The listing builds one solid part. Answer for the finished solid, in the listing's coordinates (mm). A direction names the side the tool comes from. Coordinates: 2 decimals unless noted, no trailing zeros. Loops run counter-clockwise (first coordinate to the right, second up) from the corner with the lowest first, then second, coordinate; pieces in that order, holes last. Notation, with made-up numbers: (43.5, 78) - (54.5, 78) arc R24 cw to (54.5, 113) - close; hole circle Ø4 at (-40, 81.25). An arc over 180 degrees is marked (long way). One line per question, with ' | ' between items.
from build123d import *

# Parameters (mm, degrees)
SKETCH1_W           = 28
SKETCH1_H           = 24
BOSS_EXTRUDE1_DEPTH = 39
SKETCH2_W           = 23
SKETCH2_H           = 32.5
SKETCH2_H_2         = 1.5
CUT_EXTRUDE1_DEPTH  = 25
CUT_EXTRUDE2_REACH  = 41
SKETCH3_R           = 5.175
CUT_EXTRUDE3_REACH  = 41
SKETCH4_R           = 1.75
FILLET1_R           = 3
SKETCH5_R           = 3.1
SKETCH5_R_2         = 1.75
BOSS_EXTRUDE2_DEPTH = 1


with BuildPart() as part:
    # Sketch1 → Boss-Extrude1 (new body)
    with BuildSketch(Plane.XY):
        with Locations((14, 12)):
            Rectangle(SKETCH1_W, SKETCH1_H)
    extrude(amount=BOSS_EXTRUDE1_DEPTH)

    # Sketch2 → Cut-Extrude1 (cut, through all)
    with BuildSketch(Plane(origin=(0, 24, 0), x_dir=(1, 0, 0), z_dir=(0, 1, 0))):
        with Locations((14, -20.25)):
            Rectangle(SKETCH2_W, SKETCH2_H)
        with Locations((14, -0.75)):
            Rectangle(SKETCH2_W, SKETCH2_H_2)
    extrude(amount=-CUT_EXTRUDE1_DEPTH, mode=Mode.SUBTRACT)

    # Sketch3 → Cut-Extrude2 (cut, up to next)
    with BuildSketch(Plane(origin=(0, 0, 0), x_dir=(-1, 0, 0), z_dir=(0, 0, -1)), mode=Mode.PRIVATE) as cut_extrude2_sk1:
        with Locations((-14, 12)):
            Circle(SKETCH3_R)
    cut_extrude2_tool1 = extrude(cut_extrude2_sk1.sketch, amount=-CUT_EXTRUDE2_REACH, mode=Mode.PRIVATE) & part.part
    add(cut_extrude2_tool1.solids().sort_by_distance((14, 12, 0))[0], mode=Mode.SUBTRACT)

    # Sketch4 → Cut-Extrude3 (cut, up to next)
    with BuildSketch(Plane.XY.offset(39), mode=Mode.PRIVATE) as cut_extrude3_sk1:
        with Locations((14, 12)):
            Circle(SKETCH4_R)
    cut_extrude3_tool1 = extrude(cut_extrude3_sk1.sketch, amount=-CUT_EXTRUDE3_REACH, mode=Mode.PRIVATE) & part.part
    add(cut_extrude3_tool1.solids().sort_by_distance((14, 12, 39))[0], mode=Mode.SUBTRACT)

    # Fillet1
    fillet1_edges = [part.edges().sort_by_distance(p)[0] for p in [
        (28, 12, 39),
        (0, 12, 39),
    ]]
    fillet(fillet1_edges, radius=FILLET1_R)

    # Sketch5 → Boss-Extrude2 (add)
    with BuildSketch(Plane.XY.offset(39)):
        with Locations((14, 12)):
            Circle(SKETCH5_R)
        with Locations((14, 12)):
            Circle(SKETCH5_R_2, mode=Mode.SUBTRACT)
    extrude(amount=BOSS_EXTRUDE2_DEPTH)


solid = part.part
Item 1: The mould has two halves that part along Z. Classify faces 1 (the face through (1, 12, 0)), 2 (the face through (14, 18, 4)), 3 (the face through (25.5, 12, 1)): pulls with the +Z half, pulls with the -Z half, needs draft (parallel to the pull), parting line crosses it, or undercut.
Taken from the geometry:
face 1: pulls with the -Z half | face 2: undercut | face 3: needs draft
Item 2: Find section C-C, the plane y = 5.75. Write down the section's boundary in (x, z).
Taken from the geometry:
outline: (0, 0) - (2.5, 0) - (2.5, 1.5) - (25.5, 1.5) - (25.5, 0) - (28, 0) - (28, 36) arc R3 ccw to (25, 39) - (3, 39) arc R3 ccw to (0, 36) - close; hole (2.5, 4) - (25.5, 4) - (25.5, 36.5) - (2.5, 36.5) - close
Item 3: Find section A-A, the plane z = 17.5. Write down the section's boundary in (x, y).
Taken from the geometry:
outline: (0, 0) - (2.5, 0) - (2.5, 24) - (0, 24) - close; (25.5, 0) - (28, 0) - (28, 24) - (25.5, 24) - close
Item 4: Find section D-D, the plane x = 14. Write down the section's boundary in (y, z) (3 decimals).
Taken from the geometry:
outline: (0, 1.5) - (6.825, 1.5) - (6.825, 4) - (0, 4) - close; (0, 36.5) - (10.25, 36.5) - (10.25, 40) - (8.9, 40) - (8.9, 39) - (0, 39) - close; (13.75, 36.5) - (24, 36.5) - (24, 39) - (15.1, 39) - (15.1, 40) - (13.75, 40) - close; (17.175, 1.5) - (24, 1.5) - (24, 4) - (17.175, 4) - close
Item 5: Each of these flat-tipped pins is pushed along its axis until it touches: pin 1 Ø12 at (x, y) = (13.5, 11.5) entering from -Z; pin 2 Ø4 at (x, y) = (14, 12) entering from -Z; pin 3 Ø1.5 at (x, y) = (18, 5) entering from +Z. Where does it stop, or does it pass through?
Taken from the geometry:
pin 1: stops at z = 1.5 | pin 2: stops at z = 36.5 | pin 3: stops at z = 39
Item 6: Find section B-B, the plane x = 24. Write down the section's boundary in (y, z), plus the area to 3 significant figures.
Taken from the geometry:
outline: (0, 1.5) - (24, 1.5) - (24, 4) - (0, 4) - close; (0, 36.5) - (24, 36.5) - (24, 39) - (0, 39) - close | area: 120 mm2
Item 7: Which of the six approach directions +Z, -Z, +X, -X, +Y, -Y give full straight-line access (tool end or side, diameter ignored) to faces 4 (the face through (11.72, 14.1, 39.49)), 5 (the face through (25.5, 12, 20)), 6 (the face through (1, 24, 19)), 7 (the face through (14, 18, 1.5)), 8 (the face through (14.67, 17.13, 2.73))?
Taken from the geometry:
face 4: +Z | face 5: +Y, -Y | face 6: +Z, -Z, +X, -X, +Y | face 7: -Z, +Y, -Y | face 8: -Z
Item 8: Find the intervals of material crossed by line 1 (X direction, y = 10, z = 8); line 2 (Y direction, x = 14, z = 38.2); line 3 (Z direction, x = 21, y = 17.5), in increasing order. Write a range as [from, to].
Taken from the geometry:
line 1: x = [0, 2.5], [25.5, 28] | line 2: y = [0, 10.25], [13.75, 24] | line 3: z = [1.5, 4], [36.5, 39]
